Source: CAD feature listing. Evaluate the final solid. Frame: model axes, mm. A direction names the side the tool comes from. Coordinates: 2 decimals unless noted, no trailing zeros. Write each loop counter-clockwise with the first axis right and the second up, starting at its lowest first coordinate (ties: lowest second). Pieces come first, ordered by that corner, then holes. Notation, with made-up numbers: (-4, 84.5) - (48, 84.5) arc R30 cw to (48, 107.5) - close; hole circle Ø8 at (-1.75, -31.75). An arc over 180 degrees is marked (long way). One line per question, with ' | ' between items.
Autodesk Inventor part; units mm, degrees
ref_plane "YZ Plane" through (0, 0, 0) normal (1, 0, 0) x (0, 1, 0)
ref_plane "XZ Plane" through (0, 0, 0) normal (0, 1, 0) x (-1, 0, 0)
ref_plane "XY Plane" through (0, 0, 0) normal (0, 0, 1) x (1, 0, 0)
sketch "Sketch1" plane through (0, 0, 0) normal (0, 1, 0) x (-1, 0, 0)
  line L0 (37, 0) -> (0, 0)
  line L1 (0, 0) -> (-3.25, -15)
  line L2 (-3.25, -15) -> (3.25, -15)
  line L3 (3.25, -15) -> (3.25, -8.5)
  line L4 (3.25, -8.5) -> (33.75, -8.5)
  line L5 (33.75, -8.5) -> (33.75, -15)
  line L6 (33.75, -15) -> (40.25, -15)
  line L7 (40.25, -15) -> (37, 0)
  line L8 (37, 0) -> (47, 0)
  line L9 (47, 0) -> (47, -20)
  line L10 (47, -20) -> (-10, -20)
  line L11 (-10, -20) -> (-10, 0)
  line L12 (-10, 0) -> (0, 0)
  dimension "d1" = 20
  dimension "d5" = 10
  dimension "d6" = 10
extrude "Extrusion1" add sketch "Sketch1" along normal blind 300 contours L8 L9 L10 L11 L12 L1 L2 L3 L4 L5 L6 L7
sketch "Sketch2" plane through (10, 0, -20) normal (0, 0, -1) x (-1, 0, 0)
  line L0 (0, 0) -> (57, 0)
  line L1 (57, 0) -> (57, 300)
  line L2 (0, 300) -> (57, 300)
  line L3 (0, 0) -> (0, 300)
  line L4 (43.75, 0) -> (13.25, 0)
  line L5 (28.5, 0) -> (28.5, 300)
  line L6 (43.75, 300) -> (13.25, 300)
  line L7 (0, 52.5) -> (57, 52.5)
  line L8 (57, 52.5) -> (57, 247.5)
  line L9 (57, 247.5) -> (0, 247.5)
  line L10 (0, 247.5) -> (0, 52.5)
  line L11 (0, 52.5) -> (57, 247.5) construction
  line L12 (57, 52.5) -> (0, 247.5) construction
  circle A0 centre (28.5, 150) radius 3.1
  line L13 (28.5, 52.5) -> (28.5, 82.5)
  circle A1 centre (28.5, 82.5) radius 3.1
  line L14 (28.5, 247.5) -> (28.5, 217.5)
  circle A2 centre (28.5, 217.5) radius 3.1
  point P0 (10, 0)
  dimension "d7" = 195
  dimension "d8" = 6.2
  dimension "d9" = 30
  dimension "d10" = 6.2
  dimension "d11" = 30
  dimension "d12" = 6.2
extrude "Extrusion2" cut sketch "Sketch2" against normal up to surface (11.5 mm away) contours A1 L5 | L5 A1 | A2 L5 | L5 A2 | A0 L5 | L5 A0
sketch "Sketch4" plane through (-33.75, 0, -8.5) normal (0, 0, 1) x (1, 0, 0)
  circle A0 centre (15.25, 217.5) radius 3.1
  circle A1 centre (15.25, 82.5) radius 3.1
  circle A2 centre (15.25, 150) radius 3.1
  line L0 (0, 0) -> (30.5, 0)
  line L1 (30.5, 0) -> (30.5, 300)
  line L2 (0, 300) -> (30.5, 300)
  line L3 (0, 0) -> (0, 300)
  circle A3 centre (15.25, 82.5) radius 3.1
  circle A4 centre (15.25, 82.5) radius 5
  circle A5 centre (15.25, 150) radius 5
  circle A6 centre (15.25, 217.5) radius 5
  point P0 (33.75, 0)
  dimension "d15" = 10
  dimension "d16" = 10
  dimension "d17" = 10
extrude "Extrusion3" cut sketch "Sketch4" against normal blind 6 contours A4 | A5 | A6
sketch "Sketch5" plane through (-33.75, 0, -8.5) normal (0, 0, 1) x (1, 0, 0)
  line L0 (43.75, 0) -> (-13.25, 0)
  line L1 (15.25, 0) -> (15.25, 10)
  line L2 (43.75, 300) -> (-13.25, 300)
  line L3 (15.25, 300) -> (15.25, 290)
  circle A0 centre (15.25, 290) radius 2.5
  circle A1 centre (15.25, 10) radius 2.5
  point P0 (33.75, 0)
  dimension "d20" = 10
  dimension "d21" = 10
  dimension "d22" = 5
  dimension "d23" = 5
extrude "Extrusion4" cut sketch "Sketch5" against normal up to surface (11.5 mm away)
thread "Thread1"
thread "Thread2"
properties part number "uchwyt_szyny" material "Aluminum 6061"
Item 1: Cut plane C-C on y = 43. Return loops of the section in (x, z).
Check sheet entries:
outline: (-47, -20) - (10, -20) - (10, 0) - (0, 0) - (3.25, -15) - (-3.25, -15) - (-3.25, -8.5) - (-33.75, -8.5) - (-33.75, -15) - (-40.25, -15) - (-37, 0) - (-47, 0) - close
Item 2: Access query for faces 4 (the face through (0, 148, -15)), 5 (the face through (-18.096, 153.074, -17.288)), 6 (the face through (-3.25, 148, -12)), 7 (the face through (-21, 215, -14.5)). Directions: +Z, -Z, +X, -X, +Y, -Y. A direction counts if a zero-diameter tool reaches every point of the face in a straight line with its end or side. Return the directions, or none.
Check sheet entries:
face 4: +Y, -Y | face 5: +Z, -Z | face 6: +Z, +Y, -Y | face 7: +Z
Item 3: Ray query, line 1 along Y through (x, z) = (-18.5, -11.25); line 2 along Y through (x, z) = (-18.5, -17.5); line 3 along X through (y, z) = (217.5, -16.15). Return the intervals inside material, ascending. Write a range as [from, to].
Check sheet entries:
line 1: [0, 7.5], [12.5, 77.5], [87.5, 145], [155, 212.5], [222.5, 287.5], [292.5, 300] | line 2: [0, 7.5], [12.5, 79.4], [85.6, 146.9], [153.1, 214.4], [220.6, 287.5], [292.5, 300] | line 3: [-47, -21.6], [-15.4, 10]
Item 4: Pin query (flat end, axial travel): pin 1 Ø1 at (x, y) = (-9.5, 97) entering from +Z; pin 2 Ø5 at (x, y) = (-18, 148.5) entering from +Z. Return the tip coordinate at first contact, or that it passes through.
Check sheet entries:
pin 1: z = -8.5 | pin 2: z = -14.5
Item 5: Mould query, pull axis Y, two halves, no side actions, for faces 1 (the face through (-18, 300, -12)), 2 (the face through (-38.648, 147.9, -7.605)), 3 (the face through (-17.828, 214.474, -17.288)). Classes: pulls with the +Y half, pulls with the -Y half, needs draft (parallel to the pull), parting line crosses it, or undercut.
Check sheet entries:
face 1: pulls with the +Y half | face 2: needs draft | face 3: undercut
Item 6: Cut plane A-A on y = 82.5. Return loops of the section in (x, z).
Check sheet entries:
outline: (-47, -20) - (-21.6, -20) - (-21.6, -14.5) - (-23.5, -14.5) - (-23.5, -8.5) - (-33.75, -8.5) - (-33.75, -15) - (-40.25, -15) - (-37, 0) - (-47, 0) - close; (-15.4, -20) - (10, -20) - (10, 0) - (0, 0) - (3.25, -15) - (-3.25, -15) - (-3.25, -8.5) - (-13.5, -8.5) - (-13.5, -14.5) - (-15.4, -14.5) - close
Item 7: Cut plane B-B on z = -11.75. Return loops of the section in (x, y).
Check sheet entries:
outline: (-47, 0) - (-39.55, 0) - (-39.55, 300) - (-47, 300) - close; (-33.75, 0) - (-3.25, 0) - (-3.25, 300) - (-33.75, 300) - close; (2.55, 0) - (10, 0) - (10, 300) - (2.55, 300) - close; hole circle Ø10 at (-18.5, 82.5); hole circle Ø10 at (-18.5, 150); hole circle Ø10 at (-18.5, 217.5); hole circle Ø5 at (-18.5, 10); hole circle Ø5 at (-18.5, 290)
